Work out the finished part from the listing and answer in its coordinate system (mm). A direction names the side the tool comes from. Coordinates: 2 decimals unless noted, no trailing zeros. Order: outer loops, then holes, each group sorted by start corner. A loop starts at its lowest first (then second) coordinate and runs counter-clockwise, first axis right, second up. Notation, with made-up numbers: (11, 40) -> (70, 40) arc R16 ccw to (70, 49) -> close; hole circle Ø8 at (7.25, 61). An arc over 180 degrees is marked (long way). Write item = value, one per line. Start each with the question number.
Q1. Flat-ended cylindrical pins translate along their axes: pin 1 (1.5 mm diameter, centred on x = -27, y = 15.5, fed in from -Z); pin 2 (5 mm diameter, centred on y = -23.5, z = 17.5, fed in from +X); pin 3 (6 mm diameter, centred on y = 6.5, z = 12, fed in from -X); pin 4 (18.5 mm diameter, centred on x = 0, y = 0, fed in from -Z). Find the tip coordinate at first contact, or state that the pin passes through.
Q2. The part is cut by section C-C, the plane z = 8.5. Determine the outline of the cut face in (x, y).
Q3. Straight lines are drawn through the part: L1, parallel to Y at x = 0, z = 16.75; L2, parallel to X at y = 15.5, z = 5.75; L3, parallel to Y at x = -2, z = 10.5. For each, find the intervals that lie inside material, in ascending order. Write a range as from..to.
Q4. For a pull along X with two mould halves and no side action, classify faces 3 (the flat face through (-26, 15, 6.312)), 4 (the cylindrical face through (28.37, 14.56, 3.11)), 5 (the cylindrical face through (17.535, 33.713, 9.86)), 6 (the flat face through (-9, -8, 20)) as +X half, -X half, draft (parallel to the pull), parting line (faces both ways), or undercut.
Q5. Which of the six approach directions +Z, -Z, +X, -X, +Y, -Y give full straight-line access (tool end or side, diameter ignored) to faces 1 (the cylindrical face through (-23.863, 14.097, 3.112)), 2 (the cylindrical face through (-1.5, -11.4, 9.9))?
Q6. The part is cut by section A-A, the plane y = 0. Determine the outline of the cut face in (x, z), plus the area to 3 significant figures.
Q7. The part is cut by section B-B, the plane x = -4.5. Determine the outline of the cut face in (y, z).
Q8. The part is cut by section D-D, the plane z = 4.5. Determine the outline of the cut face in (x, y).
Autodesk Fusion 360 part; units mm, degrees
sketch "Sketch1" plane through (0, 0, 0) normal (0, 0, 1) x (1, 0, 0)
  circle A0 centre (0, 0) radius 11.5
  circle A1 centre (0, 0) radius 22.5
  circle A2 centre (0, 0) radius 38
  dimension "d1" = 45
  dimension "d2" = 23
  dimension "d3" = 76
extrude "Extrude1" add sketch "Sketch1" along normal blind 20 contours A1
sketch "Sketch2" plane through (0, 0, 0) normal (0, 0, 1) x (1, 0, 0)
  circle A0 centre (0.2654, -30.1553) radius 2.5
  dimension "d8" = 5
extrude "Extrude4" add sketch "Sketch1" along normal blind 20 contours A1 | A2
extrude "Extrude5" cut sketch "Sketch2" along normal blind 6.312
pattern_circular "C-Pattern2" count 3 over 360 about axis through (0, 0, 20) along (0, 0, 1) of "Extrude5"
Model answer:
q1.pin_1 = 6.31
q1.pin_2 = 31.67
q1.pin_3 = -37.84
q1.pin_4 = through
q2.outline = circle Ø76 at (0, 0); hole circle Ø23 at (0, 0)
q3.L1 = -38..-11.5, 11.5..38
q3.L2 = -34.7..-28.66, -23.83..23.49, 28.48..34.7
q3.L3 = -37.95..-11.32, 11.32..37.95
q4.face_3 = undercut
q4.face_4 = undercut
q4.face_5 = parting line
q4.face_6 = draft
q5.face_1 = -Z
q5.face_2 = +Z, -Z
q6.outline = (-38, 0) -> (-11.5, 0) -> (-11.5, 20) -> (-38, 20) -> close; (11.5, 0) -> (38, 0) -> (38, 20) -> (11.5, 20) -> close
q6.area = 1,060 mm2
q7.outline = (-37.73, 0) -> (-10.58, 0) -> (-10.58, 20) -> (-37.73, 20) -> close; (10.58, 0) -> (37.73, 0) -> (37.73, 20) -> (10.58, 20) -> close
q8.outline = circle Ø76 at (0, 0); hole circle Ø5 at (-26.25, 14.85); hole circle Ø23 at (0, 0); hole circle Ø5 at (0.27, -30.16); hole circle Ø5 at (25.98, 15.31)
